Geometry: see drawing. Coordinates: mm, zero at the bounding-box minimum. A direction names the side the tool comes from. Give positions to 0.01 mm unless a question says otherwise; leave off trailing zeros. Write each loop counter-clockwise with the first axis right and the second up, starting at its lowest first coordinate (ties: lowest second). Pieces come first, ordered by that corner, then holes. Notation, with made-up numbers: (8.5, 27.25) -> (36.5, 27.25) arc R33 ccw to (36.5, 59.25) -> close; hole circle Ø10 at (6, 36). An arc over 180 degrees is marked (long way). Use one line per item in the form item = value. Start each with the question number.
(1) Cut plane A-A, the plane x = 15.5. Output: boundary loops of the cut face in (y, z).
(2) Cut plane C-C, the plane y = 4.5. Count the separate pieces of the cut face and the enclosed holes in it, and give its area (3 significant figures).
(3) Draft query along X for the marked faces 1, 2, 3 and 4. Return one class per face: pulls with the +X half, pulls with the -X half, needs draft (parallel to the pull), parting line crosses it, or undercut.
(4) Cut plane B-B, the plane z = 9.5. Output: boundary loops of the cut face in (x, y).
(5) Cut plane D-D, the plane x = 47. Output: boundary loops of the cut face in (y, z), and give its area (3 significant figures).
(6) Set-up query: the marked faces 5 and 6. Return all of +Z, -Z, +X, -X, +Y, -Y with unobstructed straight access to the full face (end or side cutting, diameter ignored); none if empty.
(7) First-contact query: P1, Ø4, axis at y = 4.5, z = 15.5, coming from the -X side; P2, Ø5.5, axis at x = 60, y = 4.5, coming from the -Z side. Flat tips, straight axial feed; report the tip coordinate or a pass-through.
(8) Material intervals for line 1 along X through (y, z) = (6.75, 16); line 2 along Z through (x, y) = (19.5, 1.5); line 3 along X through (y, z) = (9.5, 10), sorted ascending. Write a range as from..to.
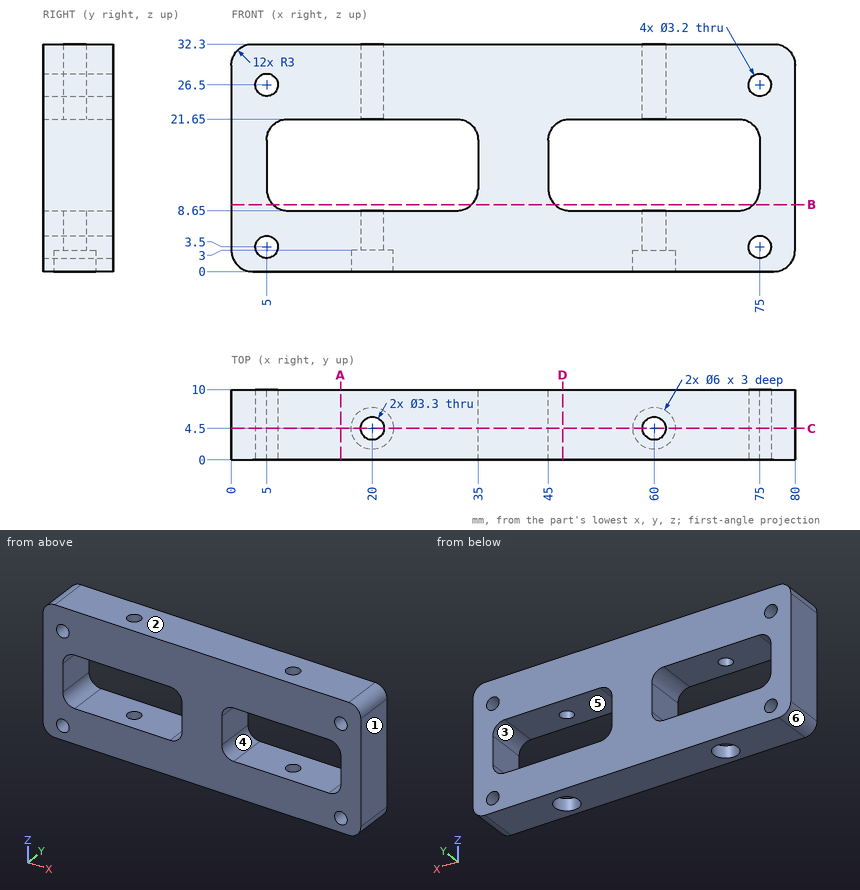
Geometry says:
q1.outline = (0, 0) -> (10, 0) -> (10, 8.65) -> (0, 8.65) -> close; (0, 21.65) -> (10, 21.65) -> (10, 32.3) -> (0, 32.3) -> close
q2.separate_pieces = 3
q2.enclosed_holes = 4
q2.area = 1,640 mm^2
q3.face_1 = pulls with the +X half
q3.face_2 = needs draft
q3.face_3 = undercut
q3.face_4 = undercut
q4.outline = (0, 0) -> (5.91, 0) -> (5.91, 10) -> (0, 10) -> close; (34.09, 0) -> (45.91, 0) -> (45.91, 10) -> (34.09, 10) -> close; (74.09, 0) -> (80, 0) -> (80, 10) -> (74.09, 10) -> close
q5.outline = (0, 0) -> (10, 0) -> (10, 8.82) -> (0, 8.82) -> close; (0, 21.48) -> (10, 21.48) -> (10, 32.3) -> (0, 32.3) -> close
q5.area = 196 mm^2
q6.face_5 = +Y, -Y
q6.face_6 = -Z, -X, +Y, -Y
q7.P1 = 0
q7.P2 = 3
q8.line_1 = 0..5, 35..45, 75..80
q8.line_2 = 0..8.65, 21.65..32.3
q8.line_3 = 0..5.49, 34.51..45.49, 74.51..80
